from build123d import *

# Parameters (mm, degrees)
F1_DEPTH    = 40
F2_W        = 38.8704487759
F2_H        = 36
F3_DEPTH    = 25
F4_R        = 7.5
F5_R        = 2
F6_T1_DEPTH = 16.8824680596
F6_T3_DEPTH = 16.8824680596
F7_R        = 5


# Not quite as in the source:
# - a fillet or chamfer that OpenCascade refuses, or shapes differently, is made with other operations: its cross-section is extruded or revolved along the edge and cut away or added


with BuildPart() as f1:
    # F0 (on Front) → F1 (new body)
    with BuildSketch(Plane.XZ):
        with BuildLine():
            Line((-48, 0), (-58, 0))
            Line((-58, 0), (-58, 5))
            Line((-58, 5), (-60, 5))
            Line((-60, 5), (-60, -2))
            Line((-60, -2), (0, -2))
            Line((0, -2), (0, 0))
            ThreePointArc((0, 0), (-18.8023659823, 7.4599490238), (-38.8704487759, 10))
            Line((-38.8704487759, 10), (-40.8704487759, 10))
            Line((-40.8704487759, 10), (-44.5101511185, 0))
            Line((-44.5101511185, 0), (-46, 0))
            Line((-46, 0), (-44.1801488287, 5))
            Line((-44.1801488287, 5), (-46.1801488287, 5))
            Line((-46.1801488287, 5), (-48, 0))
        make_face()
    extrude(amount=F1_DEPTH)

    # F2 (on face) → F3 (cut)
    with BuildSketch(Plane.XY.offset(10)):
        with Locations((-19.4352243879, -20)):
            Rectangle(F2_W, F2_H)
    extrude(amount=-F3_DEPTH, mode=Mode.SUBTRACT)

    # F4
    f4_edges = [f1.edges().sort_by_distance(p)[0] for p in [
        (-48, -20, 0),
    ]]
    fillet(f4_edges, radius=F4_R)

    # F5
    f5_edges = [f1.edges().sort_by_distance(p)[0] for p in [
        (-58, -20, 0),
    ]]
    fillet(f5_edges, radius=F5_R)

    # F6: fillet of radius 5 on 2 edges, made by hand

    # F6_s2 → F6_t1 (cut)
    with BuildSketch(Plane.XZ.offset(30.5587659702)):
        with BuildLine():
            ThreePointArc((0, -2), (-0.9346139409, -0.0091871804), (-2.6330480047, 1.3880102401))
            ThreePointArc((-2.6330480047, 1.3880102401), (-1.3101118631, 0.7061689139), (0, 0))
            Line((0, 0), (0, -2))
        make_face()
    extrude(amount=F6_T1_DEPTH, mode=Mode.SUBTRACT)

    # F6_s4 → F6_t3 (cut)
    with BuildSketch(Plane.XZ.offset(-7.4412340298)):
        with BuildLine():
            ThreePointArc((0, -2), (-0.9346139409, -0.0091871804), (-2.6330480047, 1.3880102401))
            ThreePointArc((-2.6330480047, 1.3880102401), (-1.3101118631, 0.7061689139), (0, 0))
            Line((0, 0), (0, -2))
        make_face()
    extrude(amount=F6_T3_DEPTH, mode=Mode.SUBTRACT)

    # F7
    f7_edges = [f1.edges().sort_by_distance(p)[0] for p in [
        (-38.870449, -38, 4),
        (-38.870449, -2, 4),
    ]]
    fillet(f7_edges, radius=F7_R)


solid = f1.part
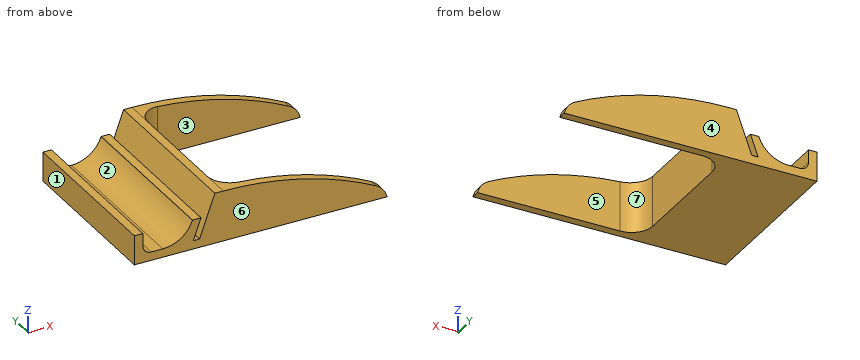
Work out the finished part from the listing and answer in its coordinate system (mm). Face numbers are marked on the shaded views. A direction names the side the tool comes from. Give positions to 0.01 mm unless a question says otherwise; leave off trailing zeros. Order: outer loops, then holes, each group sorted by start corner. A loop starts at its lowest first (then second) coordinate and runs counter-clockwise, first axis right, second up. Notation, with made-up numbers: (62.25, 49.25) - (108.25, 49.25) arc R18 cw to (108.25, 75.25) - close; hole circle Ø8 at (-3.75, 27.25). An arc over 180 degrees is marked (long way). Answer as CSV lines item,"result". Start each with the question number.
Q1. The part is cut by section C-C (z = 7.75). Write down the section's boundary in (x, y), then the cut area to 3 significant figures.
Q2. For the marked faces 1, 2 and 3, determine the directions among +Z, -Z, +X, -X, +Y, -Y from which every point of the face is accessible in a straight line to the end or side of a thin tool.
Q3. The part is cut by section B-B (y = -9). Write down the section's boundary in (x, z), then the cut area to 3 significant figures.
Q4. The mould has two halves that part along Y. Classify the marked faces 4, 5, 6 and 7: +Y half, -Y half, draft (parallel to the pull), parting line (faces both ways), or undercut.
Q5. Find the intervals of material crossed by L1, parallel to X at y = -29.5, z = 2; L2, parallel to Y at x = -22, z = 3.25; L3, parallel to X at y = -22, z = 2.25, in increasing order. Write a range as [from, to].
Q6. Given pin 1 Ø2 at (x, y) = (-58.5, -28) entering from +Z; pin 2 Ø4 at (y, z) = (-17, 8) entering from +X; pin 3 Ø0.8 at (x, y) = (-54, -10) entering from +Z; pin 4 Ø1 at (x, z) = (-37.5, 8) entering from +Y, each flat-ended and moving along its own axis, determine where each tip first touches the part or whether it passes through.
Q7. The part is cut by section A-A (x = -29.5). Write down the section's boundary in (y, z), then the cut area to 3 significant figures.
Q8. The part is cut by section D-D (x = -11). Write down the section's boundary in (y, z).
Check result:
1,outline,"(-41.69, -40) - (-19.97, -40) - (-19.97, -38) - (-33.87, -38) arc R5 cw to (-38.87, -33) - (-38.87, -7) arc R5 cw to (-33.87, -2) - (-19.97, -2) - (-19.97, 0) - (-41.69, 0) - close"
1,area,"199 mm²"
2,face 1,"+Z, -Z, -X, +Y, -Y"
2,face 2,"+Z, +Y, -Y"
2,face 3,"+Z, -Z, +X"
3,outline,"(-60, -2) - (-38.87, -2) - (-38.87, 10) - (-40.87, 10) - (-44.51, 0) - (-46, 0) - (-44.18, 5) - (-46.18, 5) - (-46.2, 4.93) arc R7.5 cw to (-53.25, 0) - (-56, 0) arc R2 cw to (-58, 2) - (-58, 5) - (-60, 5) - close"
3,area,"106 mm²"
4,face 4,"+Y half"
4,face 5,"undercut"
4,face 6,"-Y half"
4,face 7,"undercut"
5,L1,"x = [-60, -58], [-48.15, -45.27], [-43.78, -38.87]"
5,L2,"y = [-40, -38], [-2, 0]"
5,L3,"x = [-60, -58], [-47.9, -45.18], [-43.69, -38.87]"
6,pin 1,"stops at z = 5"
6,pin 2,"stops at x = -38.87"
6,pin 3,"stops at z = 0"
6,pin 4,"stops at y = 0"
7,outline,"(-40, -2) - (-38, -2) - (-38, 9.45) - (-40, 9.45) - close; (-2, -2) - (0, -2) - (0, 9.45) - (-2, 9.45) - close"
7,area,"45.8 mm²"
8,outline,"(-40, -2) - (-38, -2) - (-38, 5.02) - (-40, 5.02) - close; (-2, -2) - (0, -2) - (0, 5.02) - (-2, 5.02) - close"
